Geometry check sheet. Reference: the model listing, model coordinates, mm. A direction names the side the tool comes from. Give positions to 0.01 mm unless a question says otherwise; leave off trailing zeros. Write each loop counter-clockwise with the first axis right and the second up, starting at its lowest first coordinate (ties: lowest second). Pieces come first, ordered by that corner, then holes. Notation, with made-up numbers: M 11,25.25 L 35,25.25 A26 cw 35,53.25 Z; hole C -28.5,85.5 d1. An arc over 180 degrees is marked long. Write each question's results on one line, items separated by ' | '.
```python
from build123d import *

# Parameters (mm, degrees)
ESQUISSE1_R                                     = 4
BOSS_EXTRU_1_DEPTH                              = 11.25
ENL_V_START                                     = 4
ESQUISSE2_R                                     = 3
ENL_V_MAT_EXTRU_1_DEPTH                         = 26.824610856
CHAMBRAGE_POUR_VIS_T_TE_CYLINDRIQUE_D           = 3.4
CHAMBRAGE_POUR_VIS_T_TE_CYLINDRIQUE_CBORE_D     = 6.5
CHAMBRAGE_POUR_VIS_T_TE_CYLINDRIQUE_CBORE_DEPTH = 2
ENL_V_MAT_EXTRU_6_DEPTH                         = 2.5
CONG_3_R                                        = 4
CONG_4_R                                        = 2


with BuildPart() as part:
    # Esquisse1 → Boss.-Extru.1 (new, symmetric)
    with BuildSketch(Plane.XY):
        with BuildLine():
            Line((-12.79525785, 23), (7.20474215, 23))
            Line((7.20474215, 23), (7.20474215, 0))
            Line((7.20474215, 0), (-7.29525785, 0))
            ThreePointArc((-7.29525785, 0), (-14.72747825, 5.039915555), (-12.79525785, 13.809475019))
            Line((-12.79525785, 13.809475019), (-12.79525785, 23))
        make_face()
        with Locations(Location((-7.29525785, 8, 0), (0, 0, 180))):
            Circle(ESQUISSE1_R, mode=Mode.SUBTRACT)
    extrude(amount=BOSS_EXTRU_1_DEPTH, both=True)

    # Esquisse2 → Enlèv. mat.-Extru.1 (cut, through all)
    with BuildSketch(Plane(origin=(0, 0, 0), x_dir=(1, 0, 0), z_dir=(0, 1, 0)).offset(ENL_V_START)):
        with Locations(Location((0, 0, 0), (0, 0, 270))):
            Circle(ESQUISSE2_R)
    extrude(amount=ENL_V_MAT_EXTRU_1_DEPTH, mode=Mode.SUBTRACT)

    # Chambrage pour vis à tête cylindrique à 6 pans creux (ou vis CHC) M31 (through all)
    with Locations(Plane(origin=(7.20474215, 0, 0), x_dir=(0, 0, -1), z_dir=(1, 0, 0))):
        with Locations((0, 17)):
            CounterBoreHole(CHAMBRAGE_POUR_VIS_T_TE_CYLINDRIQUE_D / 2, CHAMBRAGE_POUR_VIS_T_TE_CYLINDRIQUE_CBORE_D / 2, CHAMBRAGE_POUR_VIS_T_TE_CYLINDRIQUE_CBORE_DEPTH)

    # Esquisse10 → Enlèv. mat.-Extru.6 (cut)
    with BuildSketch(Plane.ZY.offset(12.79525785)):
        Polygon((1.58771324, 14.25), (3.175426481, 17), (1.58771324, 19.75), (-1.58771324, 19.75), (-3.175426481, 17), (-1.58771324, 14.25), align=None)
    extrude(amount=-ENL_V_MAT_EXTRU_6_DEPTH, mode=Mode.SUBTRACT)

    # Congé3
    # the kernel refuses this fillet: 4 mm, written as the material it adds along each edge
    with BuildSketch(Plane(origin=(-12.79525785, 13.809475019, -11.25), x_dir=(0, 1, 0), z_dir=(0, 0, 1))) as cong_3_piece_1_section:
        with BuildLine():
            CenterArc((1.52196413, 4), CONG_3_R, 232.341537994, 37.658462006)
            ThreePointArc((-0.92184892, 0.833333333), (-0.444719275, 0.434593145), (0, 0))
            Line((0, 0), (1.52196413, 0))
        make_face()
    cong_3_piece_1 = extrude(amount=22.5, mode=Mode.PRIVATE)
    cong_3_piece_1 = split(cong_3_piece_1, bisect_by=Plane(origin=(-12.787909879, 14.25, -6.543416313), z_dir=(0, 1, 0)), keep=Keep.TOP, mode=Mode.PRIVATE)
    cong_3_piece_1 = split(cong_3_piece_1, bisect_by=Plane(origin=(-12.787909879, 16.719497951, -3.013478547), z_dir=(0, -0.5000000000000004, -0.8660254037844384)), keep=Keep.TOP, mode=Mode.PRIVATE)
    add(cong_3_piece_1)
    with BuildSketch(Plane(origin=(-12.79525785, 13.809475019, -11.25), x_dir=(0, 1, 0), z_dir=(0, 0, 1))) as cong_3_piece_2_section:
        with BuildLine():
            CenterArc((1.52196413, 4), CONG_3_R, 232.341537994, 37.658462006)
            ThreePointArc((-0.92184892, 0.833333333), (-0.444719275, 0.434593145), (0, 0))
            Line((0, 0), (1.52196413, 0))
        make_face()
    cong_3_piece_2 = extrude(amount=22.5, mode=Mode.PRIVATE)
    cong_3_piece_2 = split(cong_3_piece_2, bisect_by=Plane(origin=(-13.040905226, 14.25, -6.25233642), z_dir=(0, -1, 0)), keep=Keep.TOP, mode=Mode.PRIVATE)
    cong_3_piece_2 = split(cong_3_piece_2, bisect_by=Plane(origin=(-13.040905226, 15.837208914, -2.504088734), z_dir=(0, -0.5000000000000004, -0.8660254037844384)), keep=Keep.TOP, mode=Mode.PRIVATE)
    add(cong_3_piece_2)
    with BuildSketch(Plane(origin=(-12.79525785, 13.809475019, -11.25), x_dir=(0, 1, 0), z_dir=(0, 0, 1))) as cong_3_piece_3_section:
        with BuildLine():
            CenterArc((1.52196413, 4), CONG_3_R, 232.341537994, 37.658462006)
            ThreePointArc((-0.92184892, 0.833333333), (-0.444719275, 0.434593145), (0, 0))
            Line((0, 0), (1.52196413, 0))
        make_face()
    cong_3_piece_3 = extrude(amount=22.5, mode=Mode.PRIVATE)
    cong_3_piece_3 = split(cong_3_piece_3, bisect_by=Plane(origin=(-13.005461126, 14.25, 0), z_dir=(0, -1, 0)), keep=Keep.TOP, mode=Mode.PRIVATE)
    cong_3_piece_3 = split(cong_3_piece_3, bisect_by=Plane(origin=(-13.005461126, 13.176729328, -0.968060129), z_dir=(0, 0.5000000000000004, 0.8660254037844384)), keep=Keep.TOP, mode=Mode.PRIVATE)
    cong_3_piece_3 = split(cong_3_piece_3, bisect_by=Plane(origin=(-13.005461126, 13.176729328, 0.968060129), z_dir=(0, 0.49999999999999994, -0.8660254037844387)), keep=Keep.TOP, mode=Mode.PRIVATE)
    add(cong_3_piece_3)
    with BuildSketch(Plane(origin=(-12.79525785, 13.809475019, -11.25), x_dir=(0, 1, 0), z_dir=(0, 0, 1))) as cong_3_piece_4_section:
        with BuildLine():
            CenterArc((1.52196413, 4), CONG_3_R, 232.341537994, 37.658462006)
            ThreePointArc((-0.92184892, 0.833333333), (-0.444719275, 0.434593145), (0, 0))
            Line((0, 0), (1.52196413, 0))
        make_face()
    cong_3_piece_4 = extrude(amount=22.5, mode=Mode.PRIVATE)
    cong_3_piece_4 = split(cong_3_piece_4, bisect_by=Plane(origin=(-12.787909879, 14.25, 6.543416313), z_dir=(0, 1, 0)), keep=Keep.TOP, mode=Mode.PRIVATE)
    cong_3_piece_4 = split(cong_3_piece_4, bisect_by=Plane(origin=(-12.787909879, 16.719497951, 3.013478547), z_dir=(0, -0.49999999999999994, 0.8660254037844387)), keep=Keep.TOP, mode=Mode.PRIVATE)
    add(cong_3_piece_4)
    with BuildSketch(Plane(origin=(-12.79525785, 13.809475019, -11.25), x_dir=(0, 1, 0), z_dir=(0, 0, 1))) as cong_3_piece_5_section:
        with BuildLine():
            CenterArc((1.52196413, 4), CONG_3_R, 232.341537994, 37.658462006)
            ThreePointArc((-0.92184892, 0.833333333), (-0.444719275, 0.434593145), (0, 0))
            Line((0, 0), (1.52196413, 0))
        make_face()
    cong_3_piece_5 = extrude(amount=22.5, mode=Mode.PRIVATE)
    cong_3_piece_5 = split(cong_3_piece_5, bisect_by=Plane(origin=(-13.040905226, 14.25, 6.25233642), z_dir=(0, -1, 0)), keep=Keep.TOP, mode=Mode.PRIVATE)
    cong_3_piece_5 = split(cong_3_piece_5, bisect_by=Plane(origin=(-13.040905226, 15.837208914, 2.504088734), z_dir=(0, -0.49999999999999994, 0.8660254037844387)), keep=Keep.TOP, mode=Mode.PRIVATE)
    add(cong_3_piece_5)
    # the kernel refuses this fillet: 4 mm, written as the material it takes off along each edge
    with BuildSketch(Plane(origin=(7.20474215, 0, -21.25), x_dir=(-1, 0, 0), z_dir=(0, 0, 1)), Plane(origin=(-12.79525785, 23, 21.25), x_dir=(0, -1, 0), z_dir=(0, 0, -1))) as cong_3_2_piece_1:
        with BuildLine():
            CenterArc((CONG_3_R, -CONG_3_R), CONG_3_R, 90, 90)
            Line((0, -CONG_3_R), (0, 0))
            Line((0, 0), (CONG_3_R, 0))
        make_face()
    extrude(amount=42.5, mode=Mode.SUBTRACT)
    with BuildSketch(Plane(origin=(7.20474215, 23, 21.25), x_dir=(0, -1, 0), z_dir=(0, 0, -1))) as cong_3_2_piece_2:
        with BuildLine():
            CenterArc((CONG_3_R, CONG_3_R), CONG_3_R, 180, 90)
            Line((0, CONG_3_R), (0, 0))
            Line((0, 0), (CONG_3_R, 0))
        make_face()
    extrude(amount=42.5, mode=Mode.SUBTRACT)

    # Congé4
    cong_4_edges = [part.edges().sort_by_distance(p)[0] for p in [
        (-2.04525785, 0, 11.25),
        (-2.79525785, 23, -11.25),
        (-2.79525785, 23, 11.25),
        (-2.04525785, 0, -11.25),
        (-12.79525785, 17.165719575, -11.25),
        (7.20474215, 11.5, -11.25),
        (-14.475125843, 4.471615724, -11.25),
        (-11.623684975, 21.828427125, -11.25),
        (6.033169275, 1.171572875, -11.25),
        (6.033169275, 21.828427125, -11.25),
        (7.20474215, 11.5, 11.25),
        (-12.79525785, 17.165719575, 11.25),
        (-14.475125843, 4.471615724, 11.25),
        (-11.623684975, 21.828427125, 11.25),
        (6.033169275, 1.171572875, 11.25),
        (6.033169275, 21.828427125, 11.25),
        (-13.009318953, 14.040444701, -11.25),
        (-13.009318953, 14.040444701, 11.25),
    ]]
    fillet(cong_4_edges, radius=CONG_4_R)


solid = part.part
```
Q1. Section check A-A (x = -6.5). Enter the section's corners in (y, z).
Answer key:
outline: M 0,-9.25 A2 ccw 2,-11.25 L 4.08,-11.25 L 4.08,11.25 L 2,11.25 A2 ccw 0,9.25 Z; M 11.92,-11.25 L 21,-11.25 A2 ccw 23,-9.25 L 23,9.25 A2 ccw 21,11.25 L 11.92,11.25 Z; hole C 17,0 d3.4
Q2. Material ranges on probe 1 along X at (y, z) = (8, 0); probe 2 along Z at (x, y) = (-5, 17); probe 3 along X at (y, z) = (8, -8.25), recorded low to high. Write a range as [from, to].
Answer key:
probe 1: x = [-15.3, -11.3], [-3.3, -3], [3, 7.2] | probe 2: z = [-11.25, -1.7], [1.7, 11.25] | probe 3: x = [-15.3, -11.3], [-3.3, 7.2]
Q3. Depth check by flat-ended pin: P1, Ø6.5, axis at x = -7.3, y = 8, coming from the +Z side; P2, Ø3, axis at y = 16, z = 0.5, coming from the -X side; P3, Ø2, axis at x = -13, z = 1, coming from the +Y side; P4, Ø1.3, axis at x = -11.5, z = 0.5, coming from the +Y side. Enter the tip coordinate at first touch or a pass-through.
Answer key:
P1: passes through | P2: stops at x = -10.3 | P3: stops at y = 21.39 | P4: stops at y = 22.43
Q4. Section check C-C (y = 8). State how many separate pieces and enclosed holes the cut face has, then the cut area to 3 significant figures.
Answer key:
separate pieces: 2 | enclosed holes: 1 | area: 295 mm2
Q5. Access from +Z, -Z, +X, -X, +Y, -Y to the whole of each face (thin tool, end or side, straight path). Record for faces 1 (the face through (-12.194, 17.191, -10.68)), 2 (the face through (2.53, 13.37, 1.61)), 3 (the face through (-12.795, 17, -6)), 4 (the face through (-12, 19.75, 0)), 5 (the face through (-12.194, 17.191, 10.68)).
Answer key:
face 1: -Z, -X, +Y | face 2: +Y | face 3: +Z, -Z, -X, +Y | face 4: -X | face 5: +Z, -X, +Y
Q6. Release check for a two-part mould opening along Z. For faces 6 (the face through (-6.44, 16.35, 1.57)), 7 (the face through (6.219, 14.117, -1.5)), 8 (the face through (-2.71, 22.4, 10.68)), 9 (the face through (6, 21.86, 0.13)) record: released by +Z, released by -Z, zero draft, split by the parting line, or undercut.
Answer key:
face 6: undercut | face 7: undercut | face 8: released by +Z | face 9: zero draft
Q7. Section check B-B (z = -8). Enter the section's corners in (x, y).
Answer key:
outline: M -13.63,12.89 A8 ccw -7.3,0 L 3.2,0 A4 ccw 7.2,4 L 7.2,19 A4 ccw 3.2,23 L -8.8,23 A4 ccw -12.8,19 L -12.8,15.33 A4 cw Z; hole C -7.3,8 d8
Q8. Section check D-D (z = 0). Enter the section's corners in (x, y).
Answer key:
outline: M -13.63,12.89 A8 ccw -7.3,0 L 3.2,0 A4 ccw 7.2,4 L 7.2,13.75 L 5.2,13.75 L 5.2,15.3 L 3,15.3 L 3,4 L -3,4 L -3,15.3 L -10.3,15.3 L -10.3,14.25 L -12.94,14.25 A4 cw Z; M -12.72,19.75 L -10.3,19.75 L -10.3,18.7 L -3,18.7 L -3,23 L -8.8,23 A4 ccw Z; M 3,18.7 L 5.2,18.7 L 5.2,20.25 L 7,20.25 A4 ccw 3.2,23 L 3,23 Z; hole C -7.3,8 d8
